Read the model definition and answer for the solid it produces. Units are mm, in the model's axes. Face numbers are marked on the shaded views. A direction names the side the tool comes from. Coordinates: 2 decimals unless noted, no trailing zeros. Write each loop counter-clockwise with the first axis right and the second up, starting at its lowest first coordinate (ties: lowest second). Pieces come first, ordered by that corner, then holes.
(1) The part is cut by section D-D, the plane x = -15.5. Determine the outline of the cut face in (y, z), and give its area (3 significant figures).
(2) The part is cut by section A-A, the plane x = -63. Determine the outline of the cut face in (y, z), and give its area (3 significant figures).
(3) Given pin 1 (8 mm diameter, centred on x = -15.5, y = 7.5, fed in from -Z); pin 2 (1.5 mm diameter, centred on x = -16.5, z = 13, fed in from +Y); pin 3 (4 mm diameter, centred on x = -69.67, z = 54.41, fed in from +Y); pin 4 (11.5 mm diameter, centred on y = 27, z = 5.5, fed in from -X), each flat-ended and moving along its own axis, determine where each tip first touches the part or whether it passes through.
(4) The part is cut by section B-B, the plane y = 4.5. Determine the outline of the cut face in (x, z), and give its area (3 significant figures).
(5) Determine the mould class of the marked faces 1, 2, 3 and 4 for opening direction Z: pulls with the +Z half, pulls with the -Z half, needs draft (parallel to the pull), parting line crosses it, or undercut.
(6) The part is cut by section C-C, the plane z = 7. Determine the outline of the cut face in (x, y).
(7) Which of the six approach directions +Z, -Z, +X, -X, +Y, -Y give full straight-line access (tool end or side, diameter ignored) to the marked faces 5, 6, 7 and 8?
(8) Straight lines are drawn through the part: line 1 along X through (y, z) = (8.5, 12); line 2 along Z through (x, y) = (-62.5, 4); line 3 along X through (y, z) = (1, 36.5). For each, find the intervals that lie inside material, in ascending order.
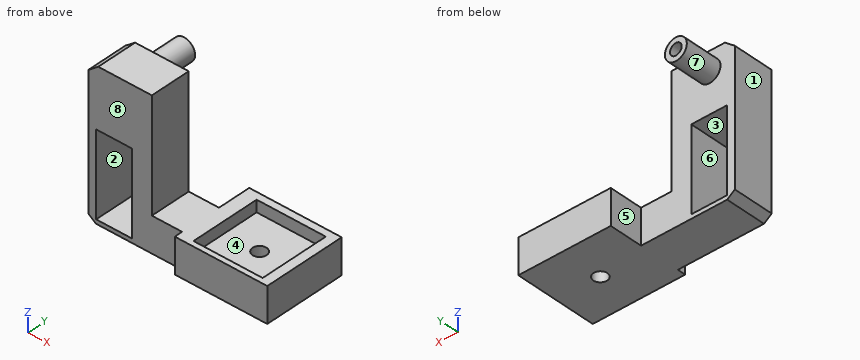
```python
from build123d import *

# Parameters (mm, degrees)
SKETCH1_W            = 55
SKETCH1_H            = 55
SKETCH1_W_2          = 30
SKETCH1_H_2          = 30
BOSS_EXTRUDE1_DEPTH  = 15
SKETCH5_W            = 70
SKETCH5_H            = 70
BOSS_EXTRUDE4_DEPTH  = 17.5
CUT_EXTRUDE1_DEPTH   = 143.483240955
SKETCH8_W            = 15.334329656
SKETCH8_H            = 35.542805721
CUT_EXTRUDE3_DEPTH   = 126.3514749
SKETCH9_R            = 4.7
BOSS_EXTRUDE5_DEPTH  = 16
SKETCH10_R           = 2.5
CUT_EXTRUDE4_DEPTH   = 10
SKETCH12_W           = 30
SKETCH12_H           = 30
BOSS_EXTRUDE6_DEPTH  = 5
SKETCH15_W           = 55
SKETCH15_H           = 15
BOSS_EXTRUDE7_DEPTH  = 18.75
SKETCH16_W           = 30
SKETCH16_H           = 30
BOSS_EXTRUDE8_DEPTH  = 10
SKETCH18_W           = 55
SKETCH18_H           = 18.75
CUT_EXTRUDE6_DEPTH   = 119.922964864
SKETCH20_W           = 15
SKETCH20_H           = 18.75
BOSS_EXTRUDE9_DEPTH  = 12
SKETCH21_W           = 12
SKETCH21_H           = 55
CUT_EXTRUDE9_DEPTH   = 119.330278287
SKETCH23_W           = 48.677589722
SKETCH23_H           = 9.375
CUT_EXTRUDE11_DEPTH  = 110.913811483
CUT_EXTRUDE13_DEPTH  = 116.802667864
SKETCH26_W           = 15
SKETCH26_H           = 9.375
CUT_EXTRUDE14_DEPTH  = 13
CUT_EXTRUDE15_DEPTH  = 111.026884691
SKETCH28_W           = 35.677589722
SKETCH28_H           = 15
BOSS_EXTRUDE10_DEPTH = 5
SKETCH22_W           = 30
SKETCH22_H           = 30
CUT_EXTRUDE16_DEPTH  = 5
SKETCH30_W           = 35.677589722
SKETCH30_H           = 5.896456585
CUT_EXTRUDE18_DEPTH  = 100.094209449
SKETCH32_W           = 15
SKETCH32_H           = 35.353543415
BOSS_EXTRUDE12_DEPTH = 4
SKETCH33_R           = 3
CUT_EXTRUDE19_DEPTH  = 102.585738893


with BuildPart() as part:
    # Sketch1 → Boss-Extrude1 (new body)
    with BuildSketch(Plane.XY):
        with Locations((-13.749602036, -10.640258422)):
            Rectangle(SKETCH1_W, SKETCH1_H)
        with Locations((-13.749602036, -10.640258422)):
            Rectangle(SKETCH1_W_2, SKETCH1_H_2, mode=Mode.SUBTRACT)
    extrude(amount=BOSS_EXTRUDE1_DEPTH)

    # Sketch12 → Boss-Extrude6 (add)
    with BuildSketch(Plane(origin=(-732.77025481, -892.317517431, 5), x_dir=(1, 0, 0), z_dir=(0, 0, 1))):
        with Locations((719.020652774, 881.677259009)):
            Rectangle(SKETCH12_W, SKETCH12_H)
    extrude(amount=-BOSS_EXTRUDE6_DEPTH)



with BuildPart() as body_2:
    # Sketch5 → Boss-Extrude4 (new body)
    with BuildSketch(Plane(origin=(0, 16.859741578, 0), x_dir=(1, 0, 0), z_dir=(0, 1, 0))):
        with Locations((-76.249602036, -35)):
            Rectangle(SKETCH5_W, SKETCH5_H)
    extrude(amount=-BOSS_EXTRUDE4_DEPTH)

    # Sketch6 → Cut-Extrude1 (cut, through all)
    with BuildSketch(Plane(origin=(0, 16.859741578, 0), x_dir=(1, 0, 0), z_dir=(0, 1, 0))):
        Polygon((-77.220552794, 0), (-111.249602036, 0), (-111.249602036, -70), (-76.249602036, -70), (-88.249602036, -61.428571429), (-88.249602036, -8.102672193), align=None)
    extrude(amount=-CUT_EXTRUDE1_DEPTH, mode=Mode.SUBTRACT)

    # Sketch8 → Cut-Extrude3 (cut, through all)
    with BuildSketch(Plane(origin=(0, 16.859741578, 0), x_dir=(1, 0, 0), z_dir=(0, 1, 0))):
        with Locations((-69.49219179, -19.543404801)):
            Rectangle(SKETCH8_W, SKETCH8_H)
    extrude(amount=-CUT_EXTRUDE3_DEPTH, mode=Mode.SUBTRACT)

    # Sketch9 → Boss-Extrude5 (add)
    with BuildSketch(Plane(origin=(0, 16.859741578, 0), x_dir=(1, 0, 0), z_dir=(0, 1, 0))):
        with Locations(Location((-69.665580404, -54.408733969, 0), (0, 0, 270))):
            Circle(SKETCH9_R)
    extrude(amount=BOSS_EXTRUDE5_DEPTH)

    # Sketch10 → Cut-Extrude4 (cut)
    with BuildSketch(Plane(origin=(0, 32.859741578, 0), x_dir=(1, 0, 0), z_dir=(0, 1, 0))):
        with Locations(Location((-69.665580404, -54.408733969, 0), (0, 0, 270))):
            Circle(SKETCH10_R)
    extrude(amount=-CUT_EXTRUDE4_DEPTH, mode=Mode.SUBTRACT)


with BuildPart() as part_1:
    add(part.part)

    add(body_2.part)  # Boss-Extrude7 merges body 2
    # Sketch15 → Boss-Extrude7 (add)
    with BuildSketch(Plane(origin=(0, 16.859741578, 0), x_dir=(1, 0, 0), z_dir=(0, 1, 0))):
        with Locations((-13.749602036, -7.5)):
            Rectangle(SKETCH15_W, SKETCH15_H)
    extrude(amount=BOSS_EXTRUDE7_DEPTH)

    # Sketch16 → Boss-Extrude8 (add)
    with BuildSketch(Plane.XY.offset(15)):
        with Locations((-13.749602036, -10.640258422)):
            Rectangle(SKETCH16_W, SKETCH16_H)
    extrude(amount=-BOSS_EXTRUDE8_DEPTH)

    # Sketch18 → Cut-Extrude6 (cut, through all)
    with BuildSketch(Plane(origin=(0, 0, 0), x_dir=(-1, 0, 0), z_dir=(0, 0, -1))):
        with Locations((13.749602036, -28.765258422)):
            Rectangle(SKETCH18_W, SKETCH18_H)
    extrude(amount=-CUT_EXTRUDE6_DEPTH, mode=Mode.SUBTRACT)

    # Sketch20 → Boss-Extrude9 (add)
    with BuildSketch(Plane.ZY.offset(41.249602036)):
        with Locations((7.5, 26.234741578)):
            Rectangle(SKETCH20_W, SKETCH20_H)
        with Locations((7.5, -10.015258422)):
            Rectangle(SKETCH20_W, SKETCH20_H)
    extrude(amount=BOSS_EXTRUDE9_DEPTH)

    # Sketch21 → Cut-Extrude9 (cut, through all)
    with BuildSketch(Plane(origin=(0, 16.859741578, 0), x_dir=(1, 0, 0), z_dir=(0, 1, 0))):
        with Locations((-47.249602036, -42.5)):
            Rectangle(SKETCH21_W, SKETCH21_H)
    extrude(amount=-CUT_EXTRUDE9_DEPTH, mode=Mode.SUBTRACT)

    # Sketch23 → Cut-Extrude11 (cut, through all)
    with BuildSketch(Plane.XY.offset(15)):
        with Locations((-28.910807175, -14.702758422)):
            Rectangle(SKETCH23_W, SKETCH23_H)
        with Locations((-28.910807175, 30.922241578)):
            Rectangle(SKETCH23_W, SKETCH23_H)
        Polygon((13.750397964, -19.390258422), (13.750397964, 35.609741578), (-4.572012314, 35.609741578), (-4.572012314, 26.234741578), (-4.572012314, -10.015258422), (-4.572012314, -19.390258422), align=None)
    extrude(amount=-CUT_EXTRUDE11_DEPTH, mode=Mode.SUBTRACT)

    # Sketch25 → Cut-Extrude13 (cut, through all)
    with BuildSketch(Plane(origin=(0, 16.859741578, 0), x_dir=(1, 0, 0), z_dir=(0, 1, 0))):
        Polygon((-80.521113565, -2.424811187), (-88.249602036, -8.102672193), (-88.249602036, -61.428571429), (-80.521113565, -66.948920336), align=None)
    extrude(amount=-CUT_EXTRUDE13_DEPTH, mode=Mode.SUBTRACT)

    # Sketch26 → Cut-Extrude14 (cut)
    with BuildSketch(Plane.ZY.offset(53.249602036)):
        with Locations((7.5, 21.547241578)):
            Rectangle(SKETCH26_W, SKETCH26_H)
    extrude(amount=-CUT_EXTRUDE14_DEPTH, mode=Mode.SUBTRACT)

    # Sketch27 → Cut-Extrude15 (cut, through all)
    with BuildSketch(Plane(origin=(0, 16.859741578, 0), x_dir=(1, 0, 0), z_dir=(0, 1, 0))):
        Polygon((-53.249602036, -70), (-53.249602036, -62.5), (-76.249602036, -62.5), (-80.521113565, -59.162729439), (-80.521113565, -66.948920336), (-76.249602036, -70), align=None)
    extrude(amount=-CUT_EXTRUDE15_DEPTH, mode=Mode.SUBTRACT)

    # Sketch28 → Boss-Extrude10 (add)
    with BuildSketch(Plane(origin=(0, 26.234741578, 0), x_dir=(1, 0, 0), z_dir=(0, 1, 0))):
        with Locations((-22.410807175, -7.5)):
            Rectangle(SKETCH28_W, SKETCH28_H)
    extrude(amount=BOSS_EXTRUDE10_DEPTH)

    # Sketch22 → Cut-Extrude16 (cut)
    with BuildSketch(Plane.XY.offset(15)):
        with Locations((-19.249602036, 13.109741578)):
            Rectangle(SKETCH22_W, SKETCH22_H)
    extrude(amount=-CUT_EXTRUDE16_DEPTH, mode=Mode.SUBTRACT)

    # Sketch30 → Cut-Extrude18 (cut, through all)
    with BuildSketch(Plane.XY.offset(15)):
        Polygon((-40.249602036, -0.640258422), (-53.249602036, -0.640258422), (-53.249602036, -10.015258422), (-40.249602036, -10.015258422), (-40.249602036, -4.118801837), align=None)
        with Locations((-22.410807175, -7.06703013)):
            Rectangle(SKETCH30_W, SKETCH30_H)
    extrude(amount=-CUT_EXTRUDE18_DEPTH, mode=Mode.SUBTRACT)

    # Sketch32 → Boss-Extrude12 (add)
    with BuildSketch(Plane(origin=(-4.572012314, 0, 0), x_dir=(0, 0, -1), z_dir=(1, 0, 0))):
        with Locations((-7.5, 13.557969871)):
            Rectangle(SKETCH32_W, SKETCH32_H)
    extrude(amount=BOSS_EXTRUDE12_DEPTH)

    # Sketch33 → Cut-Extrude19 (cut, through all)
    with BuildSketch(Plane.XY.offset(10)):
        with Locations((-19.410807175, 13.109741578)):
            Circle(SKETCH33_R)
    extrude(amount=-CUT_EXTRUDE19_DEPTH, mode=Mode.SUBTRACT)


solid = part_1.part
```
Computed:
1. outline: (-4.12, 0) - (31.23, 0) - (31.23, 15) - (28.11, 15) - (28.11, 10) - (-1.89, 10) - (-1.89, 15) - (-4.12, 15) - close
1. area: 380 mm2
2. outline: (-0.64, 0) - (16.86, 0) - (16.86, 1.77) - (-0.64, 1.77) - close; (-0.64, 37.31) - (16.86, 37.31) - (16.86, 62.5) - (-0.64, 62.5) - close
2. area: 472 mm2
3. pin 1: stops at z = 0
3. pin 2: stops at y = 31.23
3. pin 3: stops at y = 22.86
3. pin 4: stops at x = -40.25
4. outline: (-80.52, 2.42) - (-77.22, 0) - (-0.57, 0) - (-0.57, 15) - (-4.57, 15) - (-4.57, 10) - (-34.25, 10) - (-34.25, 15) - (-53.25, 15) - (-53.25, 62.5) - (-76.25, 62.5) - (-80.52, 59.16) - close; hole (-77.16, 1.77) - (-61.83, 1.77) - (-61.83, 37.31) - (-77.16, 37.31) - close
4. area: 1,790 mm2
5. face 1: needs draft
5. face 2: undercut
5. face 3: undercut
5. face 4: pulls with the +Z half
6. outline: (-80.52, -0.64) - (-77.16, -0.64) - (-77.16, 16.86) - (-80.52, 16.86) - close; (-61.83, -0.64) - (-40.25, -0.64) - (-40.25, -4.12) - (-0.57, -4.12) - (-0.57, 31.23) - (-40.25, 31.23) - (-40.25, 16.86) - (-61.83, 16.86) - close; hole circle Ø6 at (-19.41, 13.11)
7. face 5: +Z, -Z, -X, +Y
7. face 6: +Y, -Y
7. face 7: +Y
7. face 8: +Z, -Z, -X, -Y
8. line 1: x = -80.52 to -77.16, -61.83 to -34.25, -4.57 to -0.57
8. line 2: z = 0 to 1.77, 37.31 to 62.5
8. line 3: x = -80.52 to -77.16, -61.83 to -53.25
